Build history of the part. All positions in model axes, mm. Face numbers are marked on the shaded views. A direction names the side the tool comes from. Coordinates: 2 decimals unless noted, no trailing zeros. Order: outer loops, then holes, each group sorted by start corner. A loop starts at its lowest first (then second) coordinate and runs counter-clockwise, first axis right, second up. Notation, with made-up numbers: M 22,0.25 L 27,0.25 A18 ccw 27,22.25 Z; hole C 42.5,77.25 d10. An arc over 180 degrees is marked long. Use a Markdown table: item, result. Add a question column.
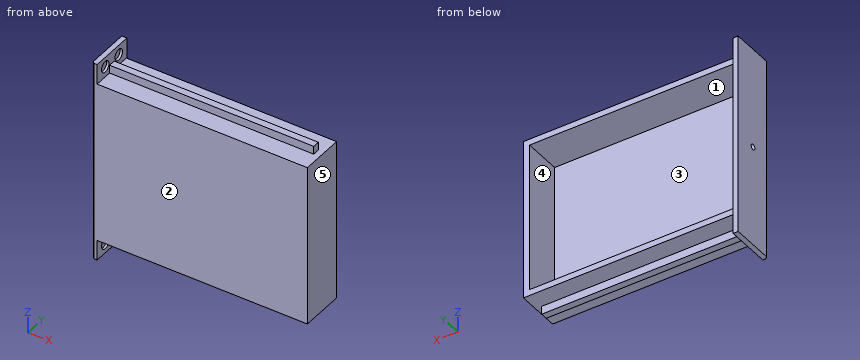
from build123d import *

# Parameters (mm, degrees)
CROQUIS1_W              = 100
CROQUIS1_H              = 22
SALIENTE_EXTRUIR1_DEPTH = 2.5
CROQUIS4_R              = 2.75
CORTAR_EXTRUIR2_DEPTH   = 1.2
SALIENTE_EXTRUIR2_DEPTH = 100.8
CROQUIS7_W              = 80
CROQUIS7_H              = 21.6
SALIENTE_EXTRUIR3_DEPTH = 3
CROQUIS8_R              = 1.4
CORTAR_EXTRUIR3_DEPTH   = 3
CHAFL_N1_SIZE           = 1


with BuildPart() as part:
    # Croquis1 → Saliente-Extruir1 (new body)
    with BuildSketch(Plane(origin=(0, 0, 0), x_dir=(0, 0, -1), z_dir=(1, 0, 0))):
        Rectangle(CROQUIS1_W, CROQUIS1_H)
    extrude(amount=SALIENTE_EXTRUIR1_DEPTH)

    # Croquis4 → Cortar-Extruir2 (cut)
    with BuildSketch(Plane(origin=(2.5, 0, 0), x_dir=(0, 0, -1), z_dir=(1, 0, 0))):
        with Locations((45.2, 5)):
            Circle(CROQUIS4_R)
        with Locations((45.2, -5)):
            Circle(CROQUIS4_R)
        with Locations((-45.2, 5)):
            Circle(CROQUIS4_R)
        with Locations((-45.2, -5)):
            Circle(CROQUIS4_R)
    extrude(amount=-CORTAR_EXTRUIR2_DEPTH, mode=Mode.SUBTRACT)

    # Croquis6 → Saliente-Extruir2 (add)
    with BuildSketch(Plane(origin=(2.5, 0, 0), x_dir=(0, 0, -1), z_dir=(1, 0, 0))):
        Polygon((-40, -11), (40, -11), (40, -1.8), (44, -1.8), (44, 1.6), (40, 1.6), (40, 10.6), (37, 10.6), (37, -8), (-37, -8), (-37, 10.6), (-40, 10.6), (-40, 1.6), (-44, 1.6), (-44, -1.8), (-40, -1.8), align=None)
    extrude(amount=SALIENTE_EXTRUIR2_DEPTH)

    # Croquis7 → Saliente-Extruir3 (add)
    with BuildSketch(Plane(origin=(103.3, 0, 0), x_dir=(0, 0, -1), z_dir=(1, 0, 0))):
        with Locations((0, -0.2)):
            Rectangle(CROQUIS7_W, CROQUIS7_H)
    extrude(amount=SALIENTE_EXTRUIR3_DEPTH)

    # Croquis8 → Cortar-Extruir3 (cut)
    with BuildSketch(Plane.ZY):
        Circle(CROQUIS8_R)
    extrude(amount=-CORTAR_EXTRUIR3_DEPTH, mode=Mode.SUBTRACT)

    # Chaflán1
    chafl_n1_edges = [part.edges().sort_by_distance(p)[0] for p in [
        (0, -11, 0),
    ]]
    chamfer(chafl_n1_edges, length=CHAFL_N1_SIZE)


solid = part.part
(1) Drop flat-ended pins along their axis: P1, Ø4, axis at x = 25.5, z = 33.5, coming from the +Y side; P2, Ø3, axis at y = 6, z = 44, coming from the +X side; P3, Ø9.5, axis at x = 29.5, y = 4.5, coming from the -Z side. Give the stop position or say it passes through.
(2) Mould opens along Z. For the marked faces 3, 4 and 5 say: released by +Z, released by -Z, zero draft, split by the parting line, or undercut.
(3) Slice it at A-A on z = 0. Give the cut face in (x, y).
(4) Slice it at B-B on y = 0. Give the cut face in (x, z), and give its area (3 significant figures).
(5) Slice it at D-D on y = 6.25. Give the cut face in (x, z).
(6) Which spindle directions (+Z, -Z, +X, -X, +Y, -Y) get a long thin tool onto all of the face, cutting with end or side? Do the marked faces 1 and 2. Say none if no direction does.
(7) Slice it at C-C on x = 26. Give the cut face in (y, z), and give its area (3 significant figures).
(8) Drill centre lines: line 1 along Y through (x, z) = (1.6, -45.2); line 2 along Z through (x, y) = (100.5, 0.25); line 3 along Z through (x, y) = (25, 2.25). Where is each one in solid material? Low to high. Write a range as from..to.
Solutions:
| question | item | result |
|---|---|---|
| 1 | P1 | y = -8 |
| 1 | P2 | x = 2.5 |
| 1 | P3 | z = -44 |
| 2 | face 3 | undercut |
| 2 | face 4 | undercut |
| 2 | face 5 | zero draft |
| 3 | outline | M 0,-10 L 1,-11 L 106.3,-11 L 106.3,10.6 L 103.3,10.6 L 103.3,-8 L 2.5,-8 L 2.5,-1.4 L 0,-1.4 Z; M 0,1.4 L 2.5,1.4 L 2.5,11 L 0,11 Z |
| 4 | outline | M 0,-50 L 2.5,-50 L 2.5,-44 L 103.3,-44 L 103.3,-40 L 106.3,-40 L 106.3,40 L 103.3,40 L 103.3,44 L 2.5,44 L 2.5,50 L 0,50 L 0,1.4 L 2.5,1.4 L 2.5,37 L 103.3,37 L 103.3,-37 L 2.5,-37 L 2.5,-1.4 L 0,-1.4 Z |
| 4 | area | 1,890 mm² |
| 5 | outline | M 0,-50 L 2.5,-50 L 2.5,-47.65 L 1.3,-47.65 L 1.3,-42.75 L 2.5,-42.75 L 2.5,-40 L 106.3,-40 L 106.3,40 L 2.5,40 L 2.5,42.75 L 1.3,42.75 L 1.3,47.65 L 2.5,47.65 L 2.5,50 L 0,50 Z; hole M 2.5,-37 L 103.3,-37 L 103.3,37 L 2.5,37 Z |
| 6 | face 1 | +Y |
| 6 | face 2 | +Z, -Z, +X, -X, -Y |
| 7 | outline | M -11,-40 L -1.8,-40 L -1.8,-44 L 1.6,-44 L 1.6,-40 L 10.6,-40 L 10.6,-37 L -8,-37 L -8,37 L 10.6,37 L 10.6,40 L 1.6,40 L 1.6,44 L -1.8,44 L -1.8,40 L -11,40 Z |
| 7 | area | 379 mm² |
| 8 | line 1 | -11..-7.75, -2.25..2.25, 7.75..11 |
| 8 | line 2 | -44..-37, 37..44 |
| 8 | line 3 | -40..-37, 37..40 |
